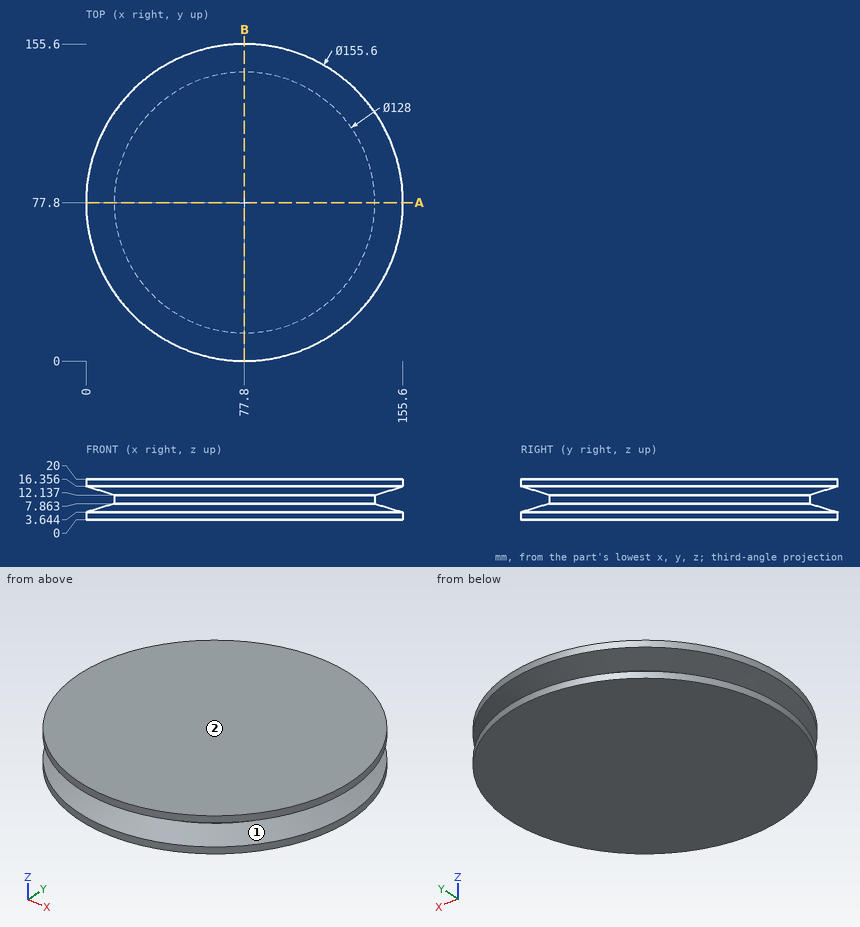
Geometry: see drawing. Coordinates: mm, zero at the bounding-box minimum. A direction names the side the tool comes from. Coordinates: 2 decimals unless noted, no trailing zeros. Loops run counter-clockwise (first coordinate to the right, second up) from the corner with the lowest first, then second, coordinate; pieces in that order, holes last. Notation, with made-up numbers: (-24.75, 54.5) - (-2.75, 54.5) arc R20 ccw to (-2.75, 64.5) - close; hole circle Ø9 at (29.25, 20.5). An arc over 180 degrees is marked (long way). Answer in a Markdown table with one row per item.
(1) Set-up query: the marked faces 1 and 2. Return all of +Z, -Z, +X, -X, +Y, -Y with unobstructed straight access to the full face (end or side cutting, diameter ignored); none if empty.
Model answer:
| item | result |
|---|---|
| face 1 | none |
| face 2 | +Z, +X, -X, +Y, -Y |
(2) Material intervals for L1, parallel to Y at x = 75.5, z = 1.5; L2, parallel to Z at x = 124, y = 28.5; L3, parallel to Y at x = 17, z = 2, sorted ascending. Write a range as from..to.
Model answer:
| item | result |
|---|---|
| L1 | y = 0.03..155.57 |
| L2 | z = 0..6.77, 13.23..20 |
| L3 | y = 29.26..126.34 |
(3) Cut plane A-A on y = 77.8. Output: boundary loops of the cut face in (x, z), plus the area to 3 significant figures.
Model answer:
| item | result |
|---|---|
| outline | (0, 0) - (155.6, 0) - (155.6, 3.64) - (141.8, 7.86) - (141.8, 12.14) - (155.6, 16.36) - (155.6, 20) - (0, 20) - (0, 16.36) - (13.8, 12.14) - (13.8, 7.86) - (0, 3.64) - close |
| area | 2,880 mm² |
(4) Pin query (flat end, axial travel): P1, Ø10, axis at y = 121.5, z = 16, coming from the -X side; P2, Ø4, axis at y = 62.5, z = 17.5, coming from the +X side; P3, Ø6, axis at x = 118.5, z = 15, coming from the -Y side (3 decimals). Return the tip coordinate at first contact, or that it passes through.
Model answer:
| item | result |
|---|---|
| P1 | stops at x = 10.32 |
| P2 | stops at x = 154.45 |
| P3 | stops at y = 9.925 |
